Read the model definition and answer for the solid it produces. Units are mm, in the model's axes. A direction names the side the tool comes from. Give positions to 0.01 mm unless a question says otherwise; leave off trailing zeros. Order: outer loops, then holes, each group sorted by start corner. A loop starts at its lowest first (then second) coordinate and runs counter-clockwise, first axis right, second up. Notation, with made-up numbers: (39, -11.75) -> (72, -11.75) arc R8 ccw to (72, -5.75) -> close; hole circle Ø6 at (81, 3.25). An arc over 180 degrees is marked (long way). One line per question, with ' | ' between items. Start each with the question number.
```python
from build123d import *

# Parameters (mm, degrees)
SKETCH_1_R               = 170
EXTRUDE_1_DEPTH          = 8
SKETCH_5_R               = 4
CUT_EXTRUDE_4_DEPTH      = 10
PATTERN_CIRCULAR_3_COUNT = 4
SKETCH_7_R               = 160
SKETCH_7_R_2             = 157
CUT_EXTRUDE_5_DEPTH      = 2
FILLET_1_R               = 0.3
SKETCH_8_R               = 15
CUT_EXTRUDE_6_DEPTH      = 10
SKETCH_10_R              = 7
CUT_EXTRUDE_7_DEPTH      = 10


with BuildPart() as part:
    # 草图1 → 凸台-拉伸1 (new body)
    with BuildSketch(Plane(origin=(0, 0, 0), x_dir=(0, 0, -1), z_dir=(1, 0, 0))):
        Circle(SKETCH_1_R)
    extrude(amount=EXTRUDE_1_DEPTH)

    # 草图5 → 切除-拉伸4 (cut)
    with BuildSketch(Plane(origin=(8, 0, 0), x_dir=(0, 0, -1), z_dir=(1, 0, 0))):
        with Locations((0, 130)):
            Circle(SKETCH_5_R)
    cut_extrude_4 = extrude(amount=-CUT_EXTRUDE_4_DEPTH, mode=Mode.SUBTRACT)

    # 阵列(圆周)3: 切除-拉伸4 ×4 about axis
    pattern_circular_3_axis = Axis((0, 0, 0), (1, 0, 0))
    for i in range(1, PATTERN_CIRCULAR_3_COUNT):
        add(cut_extrude_4.rotate(pattern_circular_3_axis, i * 360 / PATTERN_CIRCULAR_3_COUNT), mode=Mode.SUBTRACT)

    # 草图7 → 切除-拉伸5 (cut)
    with BuildSketch(Plane(origin=(8, 0, 0), x_dir=(0, 0, -1), z_dir=(1, 0, 0))):
        Circle(SKETCH_7_R)
        Circle(SKETCH_7_R_2, mode=Mode.SUBTRACT)
    extrude(amount=-CUT_EXTRUDE_5_DEPTH, mode=Mode.SUBTRACT)

    # 圆角1
    fillet_1_edges = [part.edges().sort_by_distance(p)[0] for p in [
        (0, 0, 170),
        (8, 0, 170),
    ]]
    fillet(fillet_1_edges, radius=FILLET_1_R)

    # 草图8 → 切除-拉伸6 (cut)
    with BuildSketch(Plane(origin=(8, 0, 0), x_dir=(0, 0, -1), z_dir=(1, 0, 0))):
        with Locations((45, 0)):
            Circle(SKETCH_8_R)
    extrude(amount=-CUT_EXTRUDE_6_DEPTH, mode=Mode.SUBTRACT)

    # 草图10 → 切除-拉伸7 (cut)
    with BuildSketch(Plane.ZY):
        with Locations((0, -80)):
            Circle(SKETCH_10_R)
        with Locations((0, 80)):
            Circle(SKETCH_10_R)
    extrude(amount=-CUT_EXTRUDE_7_DEPTH, mode=Mode.SUBTRACT)


solid = part.part
```
Q1. Determine the mould class of faces 3 (the cylindrical face through (3.95, -103.44, 134.91)), 4 (the flat face through (8, 51, 152)), 5 (the cylindrical face through (7.014, -156.195, 34.685)) for opening direction Y: pulls with the +Y half, pulls with the -Y half, needs draft (parallel to the pull), parting line crosses it, or undercut.
Q2. Which of the six approach directions +Z, -Z, +X, -X, +Y, -Y give full straight-line access (tool end or side, diameter ignored) to faces 1 (the flat face through (6, -118, -106)), 2 (the cylindrical face through (3.94, 86.94, -0.91))?
Q3. A cutting plane is placed at B-B, the plane z = 0. Give the number of separate pieces and of enclosed holes in the cut face, then the cut area to 3 significant figures.
Q4. Find the intervals of material crossed by line 1 (Y direction, x = 4, z = 0); line 2 (Y direction, x = 7.5, z = -118); line 3 (Y direction, x = 7, z = 14.5), in increasing order.
Q5. Given P1, Ø4, axis at x = 5, y = -63.5, coming from the +Z side; P2, Ø1.5, axis at x = 4, z = 112, coming from the -Y side, each flat-ended and moving along its own axis, determine where each tip first touches the part or whether it passes through.
Q6. A cutting plane is placed at A-A, the plane x = 3.5. Determine the outline of the cut face in (y, z), then the cut area to 3 significant figures.
Q7. A cutting plane is placed at C-C, the plane y = 0. Determine the outline of the cut face in (x, z), then the cut area to 3 significant figures.
Geometry results:
1) face 3: parting line crosses it | face 4: needs draft | face 5: undercut
2) face 1: +X | face 2: +X, -X
3) separate pieces: 5 | enclosed holes: 0 | area: 2,360 mm²
4) line 1: -170 to -134, -126 to -87, -73 to 73, 87 to 126, 134 to 170 | line 2: -122.38 to -108.06, -103.56 to 103.56, 108.06 to 122.38 | line 3: -169.38 to -159.34, -156.33 to 156.33, 159.34 to 169.38
5) P1: z = 158.49 | P2: y = -128.54
6) outline: circle Ø340 at (0, 0); hole circle Ø8 at (-130, 0); hole circle Ø14 at (-80, 0); hole circle Ø30 at (0, -45); hole circle Ø8 at (0, -130); hole circle Ø8 at (0, 130); hole circle Ø14 at (80, 0); hole circle Ø8 at (130, 0) | area: 89,600 mm²
7) outline: (0, -169.7) arc R0.3 ccw to (0.3, -170) -> (7.7, -170) arc R0.3 ccw to (8, -169.7) -> (8, -160) -> (6, -160) -> (6, -157) -> (8, -157) -> (8, -134) -> (0, -134) -> close; (0, -126) -> (8, -126) -> (8, -60) -> (0, -60) -> close; (0, -30) -> (8, -30) -> (8, 126) -> (0, 126) -> close; (0, 134) -> (8, 134) -> (8, 157) -> (6, 157) -> (6, 160) -> (8, 160) -> (8, 169.7) arc R0.3 ccw to (7.7, 170) -> (0.3, 170) arc R0.3 ccw to (0, 169.7) -> close | area: 2,340 mm²
